Part model, mm, in its own coordinate system. A direction names the side the tool comes from. Round coordinates to 2 decimals unless told otherwise and drop trailing zeros. Write each loop counter-clockwise with the first axis right and the second up, starting at its lowest first coordinate (ties: lowest second). Pieces come first, ordered by that corner, then holes. Notation, with made-up numbers: M 46.5,-33 L 94.5,-33 A32 ccw 94.5,0 Z; hole C 76,71.25 d6. An arc over 180 degrees is marked long. Use a Markdown table: item, result. Add a question column.
1) Drop flat-ended pins along their axis: P1, Ø1.6, axis at x = -3.5, y = 3.5, coming from the -Z side; P2, Ø1.6, axis at y = 0, z = -4, coming from the -X side; P3, Ø6, axis at x = -10, y = 0, coming from the -Z side. Give the stop position or say it passes through.
2) Slice it at D-D on z = -4.15. Write the cut outline in (x, y).
3) Two-plate mould, pull along Y, no slides. Class faces 3 (the face through (1, -7, -4)), 4 (the face through (1, 7, -4)), 5 (the face through (2, 0, -5)), 6 (the face through (-11.9, 0.08, -1.38)): released by +Y, released by -Y, zero draft, split by the parting line, or undercut.
4) Slice it at C-C on x = -10.5. Write the cut outline in (y, z).
5) Wall check: probe 1 along Y at (x, z) = (-10, -1.15); probe 2 along Z at (x, y) = (-11.5, -3); probe 3 along Z at (x, y) = (-2, 4.5). Give the ranges that are in metal, low to high.
6) Slice it at A-A on y = 0. Write the cut outline in (x, z), plus the area to 3 significant figures.
7) Slice it at B-B on z = -2.1. Write the cut outline in (x, y), plus the area to 3 significant figures.
8) Which spindle directions (+Z, -Z, +X, -X, +Y, -Y) get a long thin tool onto all of the face, cutting with end or side? Do faces 1 (the face through (0, 0, -4)), 2 (the face through (-6, 0, 0)). Say none if no direction does.
```python
from build123d import *

# Parameters (mm, degrees)
SKETCH2_R           = 1.89991352
BOSS_EXTRUDE1_DEPTH = 2.8
SKETCH3_W           = 8.5
SKETCH3_H           = 14
BOSS_EXTRUDE2_DEPTH = 0.2
SKETCH4_W           = 3
SKETCH4_H           = 14
BOSS_EXTRUDE3_DEPTH = 2


with BuildPart() as part:
    # Sketch2 → Boss-Extrude1 (new body)
    with BuildSketch(Plane.XY):
        with BuildLine():
            Line((3, 7), (-12.123370128, 7.000155991))
            ThreePointArc((-12.123370128, 7.000155991), (-13.999397778, -1.288e-06), (-12.123378453, -7.000160797))
            Line((-12.123378453, -7.000160797), (3, -7))
            Line((3, -7), (3, 7))
        make_face()
        with Locations((-10.000000707, 1.18e-07)):
            Circle(SKETCH2_R, mode=Mode.SUBTRACT)
    extrude(amount=-BOSS_EXTRUDE1_DEPTH)

    # Sketch3 → Boss-Extrude2 (add)
    with BuildSketch(Plane(origin=(0, 0, -2.8), x_dir=(-1, 0, 0), z_dir=(0, 0, -1))):
        with Locations((1.25, 0)):
            Rectangle(SKETCH3_W, SKETCH3_H)
    extrude(amount=BOSS_EXTRUDE2_DEPTH)

    # Sketch4 → Boss-Extrude3 (add)
    with BuildSketch(Plane(origin=(0, 0, -3), x_dir=(-1, 0, 0), z_dir=(0, 0, -1))):
        with Locations((-1.5, 0)):
            Rectangle(SKETCH4_W, SKETCH4_H)
    extrude(amount=BOSS_EXTRUDE3_DEPTH)


solid = part.part
```
Entries:
| question | item | result |
|---|---|---|
| 1 | P1 | stops at z = -3 |
| 1 | P2 | stops at x = 0 |
| 1 | P3 | stops at z = -2.8 |
| 2 | outline | M 0,-7 L 3,-7 L 3,7 L 0,7 Z |
| 3 | face 3 | released by -Y |
| 3 | face 4 | released by +Y |
| 3 | face 5 | zero draft |
| 3 | face 6 | undercut |
| 4 | outline | M -7,-2.8 L -1.83,-2.8 L -1.83,0 L -7,0 Z; M 1.83,-2.8 L 7,-2.8 L 7,0 L 1.83,0 Z |
| 5 | probe 1 | y = -7 to -1.9, 1.9 to 7 |
| 5 | probe 2 | z = -2.8 to 0 |
| 5 | probe 3 | z = -3 to 0 |
| 6 | outline | M -14,-2.8 L -11.9,-2.8 L -11.9,0 L -14,0 Z; M -8.1,-2.8 L -5.5,-2.8 L -5.5,-3 L 0,-3 L 0,-5 L 3,-5 L 3,0 L -8.1,0 Z |
| 6 | area | 44.7 mm^2 |
| 7 | outline | M -12.12,-7 L 3,-7 L 3,7 L -12.12,7 A14 ccw Z; hole C -10,0 d3.8 |
| 7 | area | 218 mm^2 |
| 8 | face 1 | -Z, -X, +Y, -Y |
| 8 | face 2 | +Z, +X, -X, +Y, -Y |
